Input: part model. Units: mm. Frame: model coordinates. A direction names the side the tool comes from. Round coordinates to 2 decimals unless told otherwise and drop trailing zeros. Order: outer loops, then holes, each group sorted by start corner. A loop starts at its lowest first (then second) coordinate and runs counter-clockwise, first axis right, second up. Notation, with made-up numbers: (78, 84.25) - (84, 84.25) arc R9 ccw to (84, 98.25) - close; hole circle Ø11 at (48.25, 28). An arc over 180 degrees is marked (long way). One line per item, written item: value. Start each with the question number.
from build123d import *

# Parameters (mm, degrees)
SKETCH1_R                   = 1.5
BOSS_EXTRUDE1_DEPTH         = 80
M2_TAPPED_HOLE1_D           = 1.6
M2_TAPPED_HOLE1_DEPTH       = 8
M2_TAPPED_HOLE1_CSINK_D     = 2.05
M2_TAPPED_HOLE1_CSINK_ANGLE = 90
M2_TAPPED_HOLE1_TIP         = 0.480688495
M2_TAPPED_HOLE2_D           = 1.6
M2_TAPPED_HOLE2_DEPTH       = 8
M2_TAPPED_HOLE2_CSINK_D     = 2.05
M2_TAPPED_HOLE2_CSINK_ANGLE = 90
M2_TAPPED_HOLE2_TIP         = 0.480688495


with BuildPart() as part:
    # Sketch1 → Boss-Extrude1 (new body)
    with BuildSketch(Plane(origin=(0, 0, 0), x_dir=(1, 0, 0), z_dir=(0, 1, 0))):
        with Locations(Location((0, 0, 0), (0, 0, 270))):
            Circle(SKETCH1_R)
    extrude(amount=BOSS_EXTRUDE1_DEPTH)

    # M2 Tapped Hole1
    with Locations(Plane(origin=(0, 80, 0), x_dir=(1, 0, 0), z_dir=(0, 1, 0))):
        with Locations((0, 0)):
            CounterSinkHole(M2_TAPPED_HOLE1_D / 2, M2_TAPPED_HOLE1_CSINK_D / 2, depth=M2_TAPPED_HOLE1_DEPTH, counter_sink_angle=M2_TAPPED_HOLE1_CSINK_ANGLE)
            with Locations((0, 0, -(M2_TAPPED_HOLE1_DEPTH + M2_TAPPED_HOLE1_TIP / 2))):  # 118° drill point
                Cone(0, M2_TAPPED_HOLE1_D / 2, M2_TAPPED_HOLE1_TIP, mode=Mode.SUBTRACT)

    # M2 Tapped Hole2
    with Locations(Plane(origin=(0, 0, 0), x_dir=(-1, 0, 0), z_dir=(0, -1, 0))):
        with Locations((0, 0)):
            CounterSinkHole(M2_TAPPED_HOLE2_D / 2, M2_TAPPED_HOLE2_CSINK_D / 2, depth=M2_TAPPED_HOLE2_DEPTH, counter_sink_angle=M2_TAPPED_HOLE2_CSINK_ANGLE)
            with Locations((0, 0, -(M2_TAPPED_HOLE2_DEPTH + M2_TAPPED_HOLE2_TIP / 2))):  # 118° drill point
                Cone(0, M2_TAPPED_HOLE2_D / 2, M2_TAPPED_HOLE2_TIP, mode=Mode.SUBTRACT)


solid = part.part
Item 1: First-contact query: pin 1 Ø1 at (x, z) = (0, 0) entering from +Y. Flat tip, straight axial feed; report the tip coordinate or a pass-through.
Item 2: Pull-direction query (X, two-part tool) for faces 1 (the face through (-0.98, 80, 0.65)), 2 (the face through (0.45, 39.44, 1.43)), 3 (the face through (0.63, 75.83, 0.49)); classes: released by +X, released by -X, zero draft, split by the parting line, or undercut.
Item 3: Reachability of faces 4 (the face through (-0.139, 71.603, -0.006)), 5 (the face through (-0.63, 4.17, 0.49)) from +Z, -Z, +X, -X, +Y, -Y: full face, straight path, thin tool, end or side. Return the list, or none.
Item 4: Line query: L1, parallel to Z at x = 0.6, y = 73.5; L2, parallel to Z at x = 0.15, y = 50; L3, parallel to X at y = 13, z = 1. Output: solid intervals per line, ascending.
Item 5: Section query A-A on y = 70. Return loops of the section in (x, z), and give its area (3 significant figures).
Geometry results:
1. pin 1: stops at y = 71.82
2. face 1: zero draft
2. face 2: split by the parting line
2. face 3: undercut
3. face 4: +Y
3. face 5: -Y
4. L1: z = -1.37 to -0.53, 0.53 to 1.37
4. L2: z = -1.49 to 1.49
4. L3: x = -1.12 to 1.12
5. outline: circle Ø3 at (0, 0)
5. area: 7.07 mm^2
